Autodesk Fusion 360 part; units mm, degrees
sketch "Sketch1" plane through (0, 0, 0) normal (0, 0, 1) x (1, 0, 0)
  line L0 (0, 0) -> (-3.7585, 6.5099)
  line L1 (-3.7585, 6.5099) -> (0, 13.0198)
  line L2 (0, 13.0198) -> (7.517, 13.0198)
  line L3 (7.517, 13.0198) -> (11.2755, 6.5099)
  line L4 (11.2755, 6.5099) -> (7.517, 0)
  line L5 (7.517, 0) -> (0, 0)
  dimension "d1" = 120
  dimension "d2" = 120
  dimension "d3" = 7.517
  dimension "d4" = 7.517
  dimension "d5" = 7.517
  dimension "d6" = 7.517
extrude "Extrude1" add sketch "Sketch1" along normal blind 14 draft 1.1
sketch "Sketch2" plane through (0, 0, 14) normal (0, 0, 1) x (-1, 0, 0)
  line L0 (0.1552, 0.2688) -> (-7.6722, 0.2688)
  line L1 (-7.6722, 0.2688) -> (-11.5859, -6.5099)
  line L2 (-11.5859, -6.5099) -> (-7.6722, -13.2886)
  line L3 (-7.6722, -13.2886) -> (0.1552, -13.2886)
  line L4 (0.1552, -13.2886) -> (4.0689, -6.5099)
  line L5 (4.0689, -6.5099) -> (0.1552, 0.2688)
  line L6 (0.1552, -13.2886) -> (-7.6722, 0.2688)
  line L7 (4.0689, -6.5099) -> (-11.5859, -6.5099)
  line L8 (-7.6722, -13.2886) -> (0.1552, 0.2688)
  circle A0 centre (-3.7585, -6.5099) radius 19
  circle A1 centre (-3.7585, -6.5099) radius 21.3499
  line L9 (5.0153, -25.9737) -> (5.8455, -26.0477)
  line L10 (4.3962, -24.2552) -> (5.1351, -23.2999)
  line L11 (-3.7585, -6.5099) -> (-3.7585, -7)
  line L12 (-13.3271, -26.7079) -> (-13.2828, -26.7025)
  line L13 (-12.3737, -24.5944) -> (-12.4136, -24.5402)
  line L14 (-3.7585, -6.5099) -> (-25.1084, -6.5099)
  line L15 (-3.7585, -6.5099) -> (-14.4334, -24.9995)
  arc A2 (-13.2585, -22.9644) -> (-14.4334, -24.9995) centre (-13.846, -23.9819) ccw
  arc A3 (-25.1084, -6.5099) -> (-22.7585, -6.5099) centre (-23.9334, -6.5099) ccw
  line L16 (-11.5859, -6.5099) -> (-0.7542, 12.2511)
  line L17 (-7.6722, -13.2886) -> (13.9911, -13.2886)
  dimension "d9" = 38
  dimension "d10" = 2.3499
extrude "Extrude2" add sketch "Sketch2" along normal blind 1.5 contours L0 L6 L8 | L0 L4 L5 A0 L16 L17 | L5 L7 L8 | L1 L6 L7 L14 L16 | L4 L6 L7 | L2 L7 L8 L14 L15 | L3 L6 L8 L15 L17 | A0 A1 L14 L15 | L14 A3 | L15 A2
extrude "Extrude3" add sketch "Sketch2" along normal blind 14.5 contours A0 A1 L14 L15 | L14 A3 | L15 A2
equation "d2 = d1"
equation "d4 = d3"
equation "d5 = d3"
equation "d6 = d3"
Build history of the part. All positions in model axes, mm. A direction names the side the tool comes from. Coordinates: 2 decimals unless noted, no trailing zeros. Order: outer loops, then holes, each group sorted by start corner. A loop starts at its lowest first (then second) coordinate and runs counter-clockwise, first axis right, second up. Notation, with made-up numbers: (59.25, -34.5) - (67.25, -34.5) arc R20 ccw to (67.25, -17.5) - close; hole circle Ø5 at (22.5, 36.5). An arc over 180 degrees is marked (long way). Put each result on its own line as item: value.
1. Saw through at C-C (z = 10). Write the cut outline in (x, y).
Answer sheet:
outline: (-3.98, 6.51) - (-0.11, -0.19) - (7.63, -0.19) - (11.5, 6.51) - (7.63, 13.21) - (-0.11, 13.21) - close
2. Drop flat-ended pins along their axis: P1, Ø12, axis at x = 4.5, y = -9.5, coming from the -Z side; P2, Ø1.6, axis at x = 1.5, z = 15, coming from the +Y side; P3, Ø4, axis at y = 3, z = 13.5, coming from the +X side. Give the stop position or say it passes through.
Answer sheet:
P1: stops at z = 14
P2: stops at y = 27.81
P3: stops at x = 25.05
3. Tool access for faces 4 (the face through (-3, 13.289, 15)), 5 (the face through (-12.337, -3.587, 21.148)), 6 (the face through (9.656, 9.852, 14.74)), 7 (the face through (23.908, 7.685, 21.148)): list every direction of +Z, -Z, +X, -X, +Y, -Y with a clear straight run to the whole face (end or side of a thin tool).
Answer sheet:
face 4: +Z, -Z, +X
face 5: +Z
face 6: +Z, -Z
face 7: +Z, -Z, +Y
4. Probe line 1 along Z through (x, y) = (-11, -2.5); line 2 along Z through (x, y) = (22, -2); line 3 along Y through (x, z) = (12, 23.25). List the from-to ranges inside material, lowest first. Write a range as [from, to].
Answer sheet:
line 1: z = [14, 15.5]
line 2: z = [14, 28.5]
line 3: y = [-13.19, -10.61], [23.63, 26.2]
5. Saw through at A-A (x = 10.5). Write the cut outline in (y, z), and give its area (3 significant figures).
Answer sheet:
outline: (-13.75, 14) - (-11.25, 14) - (-11.25, 28.5) - (-13.75, 28.5) - close; (4.63, 14) - (5.17, 0) - (7.85, 0) - (8.39, 14) - (8.39, 15.5) - (4.63, 15.5) - close; (24.27, 14) - (26.77, 14) - (26.77, 28.5) - (24.27, 28.5) - close
area: 123 mm^2
6. Saw through at B-B (y = -7.5). Write the cut outline in (x, z), and give its area (3 significant figures).
Answer sheet:
outline: (-12.35, 14) - (3.5, 14) - (3.5, 15.5) - (-9.08, 15.5) - (-9.08, 28.5) - (-12.35, 28.5) - close; (16.59, 14) - (19.87, 14) - (19.87, 28.5) - (16.59, 28.5) - close
area: 114 mm^2
7. Saw through at D-D (y = 11.5). Write the cut outline in (x, z).
Answer sheet:
outline: (-17, 14) - (-1.19, 14) - (-0.88, 0) - (8.39, 0) - (8.7, 14) - (8.7, 15.5) - (-14.57, 15.5) - (-14.57, 28.5) - (-17, 28.5) - close
8. Pull direction X, two halves, no side cores. Call faces 1 (the face through (4, 7, 0)), 2 (the face through (-14.327, -4.835, 21.148)), 3 (the face through (-2, 3, 15.5)): pulls with the +X half, pulls with the -X half, needs draft (parallel to the pull), parting line crosses it, or undercut.
Answer sheet:
face 1: needs draft
face 2: parting line crosses it
face 3: undercut
